Can you work these out from the model? Positions are in its coordinate system, mm. A direction names the side the tool comes from. Coordinates: 2 decimals unless noted, no trailing zeros. Order: outer loops, then holes, each group sorted by start corner. A loop starts at its lowest first (then second) coordinate and runs counter-clockwise, first axis right, second up. Notation, with made-up numbers: M 79,41 L 109,41 A22 cw 109,73 Z; hole C -14,43.5 d3. An arc over 180 degrees is marked long. Answer as CSV lines item,"result". Start each with the question number.
1. If we section it at C-C (y = -7): List the corners of the cut face in (x, z) for me.
2. If we section it at B-B (x = -17.5): List the corners of the cut face in (y, z) for me, plus the area to 3 significant figures.
3. If we mould it in two halves opening along X, with no side actions, what happens to faces 1 (the face through (21.506, 0.264, 2.465)), 2 (the face through (48.78, 0.15, 41.94)), 3 (the face through (-7.327, 0.154, 6.426))? For each: released by +X, released by -X, zero draft, split by the parting line, or undercut.
4. If we section it at A-A (y = 0): List the corners of the cut face in (x, z) for me, plus the area to 3 significant figures.
5. If we section it at D-D (z = 33): List the corners of the cut face in (x, y) for me, plus the area to 3 significant figures.
6. Will these pins go through, and if not, where does the flat tip stop? pin 1 (11 mm diameter, centred on x = -27.5, y = 0, fed in from -Z); pin 2 (10 mm diameter, centred on x = -1, y = -5, fed in from +Z); pin 3 (4 mm diameter, centred on y = 4.5, z = 2, fed in from -X); pin 4 (10 mm diameter, centred on x = 14.5, z = 36.5, fed in from -Y).
7. On a 3-axis mill with a long thin cutter (end or side, diameter ignored), from which of +Z, -Z, +X, -X, +Y, -Y can I reach the whole of each face in a straight line? I mean faces 4 (the face through (-33.494, 0.264, 2.465)), 5 (the face through (29.045, -0.154, 28.302)), 6 (the face through (-29.561, 0.154, 28.503)), 7 (the face through (39.966, 0, 2)), 8 (the face through (0, 11.034, 20)). Say none if no direction works.
8. I need wall thicknesses on line 1 along Y through (x, z) = (-27, 1); line 2 along X through (y, z) = (-6.75, 35.5); line 3 along Z through (x, y) = (20, 9.75). Which ranges of each line are inside material? Lowest first, please. Write a range as from..to.
```python
from build123d import *

# Parameters (mm, degrees)
F0_W          = 79.9313783646
F0_H          = 22.0680292696
F0_R          = 6
F1_DEPTH      = 5
F3_DEPTH      = 11.0340146348
F3_DEPTH_BACK = 11.0340146348
F4_T1_DEPTH   = 22.0680292696
F4_T3_DEPTH   = 22.0680292696
F4_T5_DEPTH   = 22.0680292696
F4_T7_DEPTH   = 22.0680292696
F4_T9_DEPTH   = 86.1669063659
F4_T11_DEPTH  = 86.1669063659


# Not quite as in the source:
# - a fillet or chamfer that OpenCascade refuses, or shapes differently, is made with other operations: its cross-section is extruded or revolved along the edge and cut away or added


with BuildPart() as f1:
    # F0 (on Top) → F1 (new body)
    with BuildSketch(Plane.XY):
        Rectangle(F0_W, F0_H)
        with Locations((-27.5, 0)):
            Circle(F0_R, mode=Mode.SUBTRACT)
        with Locations((27.5, 0)):
            Circle(F0_R, mode=Mode.SUBTRACT)
    extrude(amount=F1_DEPTH)

    # F2 (on Front) → F3 (join, two sides)
    with BuildSketch(Plane.XZ) as f3_sk:
        with BuildLine():
            ThreePointArc((-5.8236527257, 29.7265377594), (-27.4373325166, 34.7576861994), (-46.5960713348, 45.9561832249))
            Line((-46.5960713348, 45.9561832249), (-56.5117387286, 45.9561832249))
            ThreePointArc((-56.5117387286, 45.9561832249), (-33.1949461114, 30.0355047329), (-5.8236527257, 23.1106856026))
            Line((-5.8236527257, 23.1106856026), (-5.8236527257, 29.7265377594))
        make_face()
        with BuildLine():
            ThreePointArc((5.8236527257, 29.7265377594), (0, 29.4976123348), (-5.8236527257, 29.7265377594))
            Line((-5.8236527257, 29.7265377594), (-5.8236527257, 23.1106856026))
            ThreePointArc((-5.8236527257, 23.1106856026), (0, 22.900505574), (5.8236527257, 23.1106856026))
            Line((5.8236527257, 23.1106856026), (5.8236527257, 29.7265377594))
        make_face()
        with BuildLine():
            Line((56.5117387285, 45.9561832249), (46.5960713348, 45.9561832249))
            ThreePointArc((46.5960713348, 45.9561832249), (27.4373325166, 34.7576861994), (5.8236527257, 29.7265377594))
            Line((5.8236527257, 29.7265377594), (5.8236527257, 23.1106856026))
            ThreePointArc((5.8236527257, 23.1106856026), (33.1949461114, 30.0355047329), (56.5117387285, 45.9561832249))
        make_face()
        with BuildLine():
            ThreePointArc((5.8236527257, 23.1106856026), (0, 22.900505574), (-5.8236527257, 23.1106856026))
            Line((-5.8236527257, 23.1106856026), (-5.8236527257, 0))
            Line((-5.8236527257, 0), (5.8236527257, 0))
            Line((5.8236527257, 0), (5.8236527257, 23.1106856026))
        make_face()
    extrude(amount=F3_DEPTH)
    extrude(f3_sk.sketch, amount=-F3_DEPTH_BACK)

    # F4: fillet of radius 5 on 6 edges, made by hand

    # F4_s2 → F4_t1 (join)
    with BuildSketch(Plane.XZ.offset(-11.0340146348)):
        with BuildLine():
            ThreePointArc((10.8236527257, 5), (7.2881188197, 6.4644660941), (5.8236527257, 10))
            Line((5.8236527257, 10), (5.8236527257, 5))
            Line((5.8236527257, 5), (10.8236527257, 5))
        make_face()
    extrude(amount=F4_T1_DEPTH)

    # F4_s4 → F4_t3 (join)
    with BuildSketch(Plane.XZ.offset(-11.0340146348)):
        with BuildLine():
            ThreePointArc((10.1927990317, 23.5461016937), (7.0717020017, 21.8910349005), (5.8236527257, 18.5860589906))
            Line((5.8236527257, 18.5860589906), (5.8236527257, 23.1106856026))
            ThreePointArc((5.8236527257, 23.1106856026), (8.0111845889, 23.2987047184), (10.1927990317, 23.5461016937))
        make_face()
    extrude(amount=F4_T3_DEPTH)

    # F4_s6 → F4_t5 (join)
    with BuildSketch(Plane.XZ.offset(-11.0340146348)):
        with BuildLine():
            ThreePointArc((-5.8236527257, 18.5860589906), (-7.0717020017, 21.8910349005), (-10.1927990317, 23.5461016937))
            ThreePointArc((-10.1927990317, 23.5461016937), (-8.0111845889, 23.2987047184), (-5.8236527257, 23.1106856026))
            Line((-5.8236527257, 23.1106856026), (-5.8236527257, 18.5860589906))
        make_face()
    extrude(amount=F4_T5_DEPTH)

    # F4_s8 → F4_t7 (join)
    with BuildSketch(Plane.XZ.offset(-11.0340146348)):
        with BuildLine():
            ThreePointArc((-10.8236527257, 5), (-7.2881188197, 6.4644660941), (-5.8236527257, 10))
            Line((-5.8236527257, 10), (-5.8236527257, 5))
            Line((-5.8236527257, 5), (-10.8236527257, 5))
        make_face()
    extrude(amount=F4_T7_DEPTH)

    # F4_s10 → F4_t9 (cut)
    with BuildSketch(Plane.XZ.offset(-43.083453183)):
        with BuildLine():
            ThreePointArc((46.5960713348, 45.9561832249), (48.7794064532, 41.8686786406), (46.6679769916, 37.743571176))
            ThreePointArc((46.6679769916, 37.743571176), (51.7530210054, 41.6543073723), (56.5117387285, 45.9561832249))
            Line((56.5117387285, 45.9561832249), (46.5960713348, 45.9561832249))
        make_face()
    extrude(amount=F4_T9_DEPTH, mode=Mode.SUBTRACT)

    # F4_s12 → F4_t11 (cut)
    with BuildSketch(Plane.XZ.offset(-43.083453183)):
        with BuildLine():
            ThreePointArc((-46.5960713348, 45.9561832249), (-48.7794064532, 41.8686786406), (-46.6679769916, 37.743571176))
            ThreePointArc((-46.6679769916, 37.743571176), (-51.7530210054, 41.6543073723), (-56.5117387286, 45.9561832249))
            Line((-56.5117387286, 45.9561832249), (-46.5960713348, 45.9561832249))
        make_face()
    extrude(amount=F4_T11_DEPTH, mode=Mode.SUBTRACT)


solid = f1.part
```
Solved:
1,outline,"M -46.67,37.74 A80.79 ccw -10.19,23.55 A5 cw -5.82,18.59 L -5.82,10 A5 cw -10.82,5 L -39.97,5 L -39.97,0 L 39.97,0 L 39.97,5 L 10.82,5 A5 cw 5.82,10 L 5.82,18.59 A5 cw 10.19,23.55 A80.79 ccw 46.67,37.74 A5 ccw 46.6,45.96 A74.19 cw -46.6,45.96 A5 ccw Z"
2,outline,"M -11.03,0 L 11.03,0 L 11.03,5 L -11.03,5 Z; M -11.03,24.82 L 11.03,24.82 L 11.03,31.59 L -11.03,31.59 Z"
2,area,"260 mm²"
3,face 1,"undercut"
3,face 2,"released by +X"
3,face 3,"released by -X"
4,outline,"M -46.67,37.74 A80.79 ccw -10.19,23.55 A5 cw -5.82,18.59 L -5.82,10 A5 cw -10.82,5 L -21.5,5 L -21.5,0 L 21.5,0 L 21.5,5 L 10.82,5 A5 cw 5.82,10 L 5.82,18.59 A5 cw 10.19,23.55 A80.79 ccw 46.67,37.74 A5 ccw 46.6,45.96 A74.19 cw -46.6,45.96 A5 ccw Z; M -39.97,0 L -33.5,0 L -33.5,5 L -39.97,5 Z; M 33.5,0 L 39.97,0 L 39.97,5 L 33.5,5 Z"
4,area,"1,190 mm²"
5,outline,"M -39.11,-11.03 L -22.53,-11.03 L -22.53,11.03 L -39.11,11.03 Z; M 22.53,-11.03 L 39.11,-11.03 L 39.11,11.03 L 22.53,11.03 Z"
5,area,"732 mm²"
6,pin 1,"z = 25.95"
6,pin 2,"z = 29.74"
6,pin 3,"x = -39.97"
6,pin 4,"through"
7,face 4,"-Z"
7,face 5,"+X, +Y, -Y"
7,face 6,"-X, +Y, -Y"
7,face 7,"-Z, +X, +Y, -Y"
7,face 8,"+Z, -Z, +X, -X, +Y"
8,line 1,"-11.03..-5.98, 5.98..11.03"
8,line 2,"-43.32..-29.23, 29.23..43.32"
8,line 3,"0..5, 25.42..32.24"
